from build123d import *

# Parameters (mm, degrees)
SKETCH_1_W          = 12
SKETCH_1_H          = 8
EXTRUDE_1_DEPTH     = 100
SKETCH_2_W          = 1
SKETCH_2_H          = 4.5
CUT_EXTRUDE_1_DEPTH = 400
CHAMFER_1_SIZE      = 0.5
SKETCH_3_R          = 1.75
CUT_EXTRUDE_2_DEPTH = 400
SKETCH_4_R          = 3
CUT_EXTRUDE_3_DEPTH = 4.5


with BuildPart() as part:
    # 草图1 → 凸台-拉伸1 (new body)
    with BuildSketch(Plane.XY):
        Rectangle(SKETCH_1_W, SKETCH_1_H)
    extrude(amount=EXTRUDE_1_DEPTH)

    # 草图2 → 切除-拉伸1 (cut)
    with BuildSketch(Plane.XY.offset(100)):
        with Locations((-5.5, 1.75)):
            Rectangle(SKETCH_2_W, SKETCH_2_H)
        with Locations((5.5, 1.75)):
            Rectangle(SKETCH_2_W, SKETCH_2_H)
    extrude(amount=-CUT_EXTRUDE_1_DEPTH, mode=Mode.SUBTRACT)

    # 倒角1
    chamfer_1_edges = [part.edges().sort_by_distance(p)[0] for p in [
        (-5, 4, 50),
        (-5, -0.5, 50),
        (-6, -0.5, 50),
        (6, -0.5, 50),
        (5, 4, 50),
        (6, -4, 50),
        (-6, -4, 50),
    ]]
    chamfer(chamfer_1_edges, length=CHAMFER_1_SIZE - 0.0001)  # a hair under: the kernel refuses the full size

    # 草图3 → 切除-拉伸2 (cut)
    with BuildSketch(Plane(origin=(0, 4, 0), x_dir=(1, 0, 0), z_dir=(0, 1, 0))):
        with Locations(Location((0, -10, 0), (0, 0, 180))):
            Circle(SKETCH_3_R)
        with Locations(Location((0, -35, 0), (0, 0, 180))):
            Circle(SKETCH_3_R)
        with Locations(Location((0, -60, 0), (0, 0, 180))):
            Circle(SKETCH_3_R)
        with Locations(Location((0, -85, 0), (0, 0, 180))):
            Circle(SKETCH_3_R)
        with Locations((0, -110)):
            Circle(SKETCH_3_R)
        with Locations((0, -135)):
            Circle(SKETCH_3_R)
        with Locations((0, -160)):
            Circle(SKETCH_3_R)
        with Locations((0, -185)):
            Circle(SKETCH_3_R)
        with Locations((0, -210)):
            Circle(SKETCH_3_R)
        with Locations((0, -235)):
            Circle(SKETCH_3_R)
        with Locations((0, -260)):
            Circle(SKETCH_3_R)
        with Locations((0, -285)):
            Circle(SKETCH_3_R)
        with Locations((0, -310)):
            Circle(SKETCH_3_R)
        with Locations((0, -335)):
            Circle(SKETCH_3_R)
        with Locations((0, -360)):
            Circle(SKETCH_3_R)
        with Locations((0, -385)):
            Circle(SKETCH_3_R)
    extrude(amount=-CUT_EXTRUDE_2_DEPTH, mode=Mode.SUBTRACT)

    # 草图4 → 切除-拉伸3 (cut)
    with BuildSketch(Plane(origin=(0, 4, 0), x_dir=(1, 0, 0), z_dir=(0, 1, 0))):
        with Locations(Location((0, -10, 0), (0, 0, 180))):
            Circle(SKETCH_4_R)
        with Locations(Location((0, -35, 0), (0, 0, 180))):
            Circle(SKETCH_4_R)
        with Locations(Location((0, -60, 0), (0, 0, 180))):
            Circle(SKETCH_4_R)
        with Locations(Location((0, -85, 0), (0, 0, 180))):
            Circle(SKETCH_4_R)
        with Locations((0, -110)):
            Circle(SKETCH_4_R)
        with Locations((0, -135)):
            Circle(SKETCH_4_R)
        with Locations((0, -160)):
            Circle(SKETCH_4_R)
        with Locations((0, -185)):
            Circle(SKETCH_4_R)
        with Locations((0, -210)):
            Circle(SKETCH_4_R)
        with Locations((0, -235)):
            Circle(SKETCH_4_R)
        with Locations((0, -260)):
            Circle(SKETCH_4_R)
        with Locations((0, -285)):
            Circle(SKETCH_4_R)
        with Locations((0, -310)):
            Circle(SKETCH_4_R)
        with Locations((0, -335)):
            Circle(SKETCH_4_R)
        with Locations((0, -360)):
            Circle(SKETCH_4_R)
        with Locations((0, -385)):
            Circle(SKETCH_4_R)
    extrude(amount=-CUT_EXTRUDE_3_DEPTH, mode=Mode.SUBTRACT)


solid = part.part
Can you work these out from the model? Positions are in its coordinate system, mm. A direction names the side the tool comes from. Round coordinates to 2 decimals unless told otherwise and drop trailing zeros. Order: outer loops, then holes, each group sorted by start corner. A loop starts at its lowest first (then second) coordinate and runs counter-clockwise, first axis right, second up. Notation, with made-up numbers: (19, -28) - (44, -28) arc R18 cw to (44, -19) - close; hole circle Ø1 at (59.25, 63.25). An arc over 180 degrees is marked (long way). Answer in a Markdown table with one row per item.
(1) For P1, Ø2, axis at x = 0, z = 60, coming from the -Y side; P2, Ø5, axis at x = 0, z = 86, coming from the +Y side; P3, Ø4.5, axis at y = 2, z = 51, coming from the +X side; P4, Ø5, axis at x = 0, z = 60, coming from the +Y side, each with a flat end and sliding along its axis, tell me the tip position at first contact or that it passes through.
From the geometry:
| item | result |
|---|---|
| P1 | passes through |
| P2 | stops at y = 4 |
| P3 | stops at x = 5 |
| P4 | stops at y = -0.5 |
(2) If we mould it in two halves opening along X, with no side actions, what happens to faces 1 (the face through (0, 0, 100)), 2 (the face through (5, 1, 51)), 3 (the face through (-6, -2, 49)), 4 (the face through (-2, -0.5, 85))? For each: released by +X, released by -X, zero draft, split by the parting line, or undercut.
From the geometry:
| item | result |
|---|---|
| face 1 | zero draft |
| face 2 | released by +X |
| face 3 | released by -X |
| face 4 | undercut |
(3) Suppose I cut it at C-C, the plane x = 0. Count the separate pieces of the cut face and the enclosed holes in it, plus the area to 3 significant figures.
From the geometry:
| item | result |
|---|---|
| separate pieces | 5 |
| enclosed holes | 0 |
| area | 643 mm2 |
(4) Which directions (+Z, -Z, +X, -X, +Y, -Y) give clear straight access to the entire face, cutting with the end or side of a thin tool? Please do faces 5 (the face through (-2, -0.5, 60)), 6 (the face through (6, -2, 49)), 7 (the face through (-5, 2, 51)).
From the geometry:
| item | result |
|---|---|
| face 5 | +Y |
| face 6 | +Z, -Z, +X, +Y, -Y |
| face 7 | +Z, -Z, -X, +Y |
(5) Suppose I cut it at A-A, the plane y = 2.25. Please give me the cut outline in (x, z).
From the geometry:
| item | result |
|---|---|
| outline | (-5, 0) - (5, 0) - (5, 100) - (-5, 100) - close; hole circle Ø6 at (0, 10); hole circle Ø6 at (0, 35); hole circle Ø6 at (0, 60); hole circle Ø6 at (0, 85) |
(6) Please list where these lines run through material, in increasing order: L1, parallel to Z at x = 0, y = -1.15; L2, parallel to Z at x = -2.25, y = 3.75; L3, parallel to X at y = -1.5, z = 85. Write a range as from..to.
From the geometry:
| item | result |
|---|---|
| L1 | z = 0..8.25, 11.75..33.25, 36.75..58.25, 61.75..83.25, 86.75..100 |
| L2 | z = 0..8.02, 11.98..33.02, 36.98..58.02, 61.98..83.02, 86.98..100 |
| L3 | x = -6..-1.75, 1.75..6 |
